```python
from build123d import *

# Parameters (mm, degrees)
SKETCH1_W               = 22
SKETCH1_H               = 52
BOSS_EXTRUDE1_DEPTH     = 9
CUT_EXTRUDE1_START      = 2
SKETCH2_W               = 20.1
SKETCH2_H               = 50.1
CUT_EXTRUDE1_DEPTH      = 10
SKETCH7_R               = 0.8
CUT_EXTRUDE6_DEPTH      = 9
CUT_EXTRUDE6_DEPTH_BACK = 2
CUT_EXTRUDE7_REACH      = 3
SKETCH8_R               = 1
CUT_EXTRUDE9_REACH      = 3
SKETCH9_R               = 1
CUT_EXTRUDE10_REACH     = 3
SKETCH10_R              = 1
CUT_EXTRUDE11_REACH     = 3
SKETCH11_R              = 1
CUT_EXTRUDE12_REACH     = 3
SKETCH12_R              = 1
CUT_EXTRUDE13_REACH     = 3
SKETCH13_R              = 1
CUT_EXTRUDE14_REACH     = 3
SKETCH14_R              = 1
CUT_EXTRUDE15_REACH     = 3
SKETCH15_R              = 1
CUT_EXTRUDE16_REACH     = 3
SKETCH16_R              = 1
SKETCH18_W              = 2.91
SKETCH18_H              = 52
BOSS_EXTRUDE2_DEPTH     = 2
SKETCH18_3_W            = 2.9
SKETCH18_3_H            = 52
BOSS_EXTRUDE3_DEPTH     = 2
SKETCH19_W              = 10
SKETCH19_H              = 7
CUT_EXTRUDE17_DEPTH     = 25.9
SKETCH20_W              = 3.86
SKETCH20_H              = 9.915252407
SKETCH20_W_2            = 4.307713093
CUT_EXTRUDE18_DEPTH     = 1


with BuildPart() as part:
    # Sketch1 → Boss-Extrude1 (new body)
    with BuildSketch(Plane(origin=(0, 0, 0), x_dir=(1, 0, 0), z_dir=(0, 1, 0))):
        Rectangle(SKETCH1_W, SKETCH1_H)
    extrude(amount=BOSS_EXTRUDE1_DEPTH)

    # Sketch2 → Cut-Extrude1 (cut)
    with BuildSketch(Plane(origin=(0, 9, 0), x_dir=(1, 0, 0), z_dir=(0, 1, 0)).offset(CUT_EXTRUDE1_START)):
        Rectangle(SKETCH2_W, SKETCH2_H)
    extrude(amount=-CUT_EXTRUDE1_DEPTH, mode=Mode.SUBTRACT)

    # Sketch7 → Cut-Extrude6 (cut, two sides)
    with BuildSketch(Plane(origin=(0, 1, 0), x_dir=(1, 0, 0), z_dir=(0, 1, 0))) as cut_extrude6_sk:
        with Locations((-8.15, -23)):
            Circle(SKETCH7_R)
    extrude(amount=CUT_EXTRUDE6_DEPTH, mode=Mode.SUBTRACT)
    extrude(cut_extrude6_sk.sketch, amount=-CUT_EXTRUDE6_DEPTH_BACK, mode=Mode.SUBTRACT)

    # Sketch8 → Cut-Extrude7 (cut, up to next)
    with BuildSketch(Plane(origin=(0, 1, 0), x_dir=(1, 0, 0), z_dir=(0, 1, 0)), mode=Mode.PRIVATE) as cut_extrude7_sk1:
        with Locations((-5.75, -12.3)):
            Circle(SKETCH8_R)
    cut_extrude7_tool1 = extrude(cut_extrude7_sk1.sketch, amount=-CUT_EXTRUDE7_REACH, mode=Mode.PRIVATE) & part.part
    add(cut_extrude7_tool1.solids().sort_by_distance((-5.75, 1, 12.3))[0], mode=Mode.SUBTRACT)
    # Sketch8 → Cut-Extrude7 (cut, up to next)
    with BuildSketch(Plane(origin=(0, 1, 0), x_dir=(1, 0, 0), z_dir=(0, 1, 0)), mode=Mode.PRIVATE) as cut_extrude7_sk2:
        with Locations((5, -12.3)):
            Circle(SKETCH8_R)
    cut_extrude7_tool2 = extrude(cut_extrude7_sk2.sketch, amount=-CUT_EXTRUDE7_REACH, mode=Mode.PRIVATE) & part.part
    add(cut_extrude7_tool2.solids().sort_by_distance((5, 1, 12.3))[0], mode=Mode.SUBTRACT)

    # Sketch9 → Cut-Extrude9 (cut, up to next)
    with BuildSketch(Plane(origin=(0, 1, 0), x_dir=(1, 0, 0), z_dir=(0, 1, 0)), mode=Mode.PRIVATE) as cut_extrude9_sk1:
        with Locations((-5.75, -9.5)):
            Circle(SKETCH9_R)
    cut_extrude9_tool1 = extrude(cut_extrude9_sk1.sketch, amount=-CUT_EXTRUDE9_REACH, mode=Mode.PRIVATE) & part.part
    add(cut_extrude9_tool1.solids().sort_by_distance((-5.75, 1, 9.5))[0], mode=Mode.SUBTRACT)
    # Sketch9 → Cut-Extrude9 (cut, up to next)
    with BuildSketch(Plane(origin=(0, 1, 0), x_dir=(1, 0, 0), z_dir=(0, 1, 0)), mode=Mode.PRIVATE) as cut_extrude9_sk2:
        with Locations((5, -9.5)):
            Circle(SKETCH9_R)
    cut_extrude9_tool2 = extrude(cut_extrude9_sk2.sketch, amount=-CUT_EXTRUDE9_REACH, mode=Mode.PRIVATE) & part.part
    add(cut_extrude9_tool2.solids().sort_by_distance((5, 1, 9.5))[0], mode=Mode.SUBTRACT)

    # Sketch10 → Cut-Extrude10 (cut, up to next)
    with BuildSketch(Plane(origin=(0, 1, 0), x_dir=(1, 0, 0), z_dir=(0, 1, 0)), mode=Mode.PRIVATE) as cut_extrude10_sk1:
        with Locations((-5.75, -6.8)):
            Circle(SKETCH10_R)
    cut_extrude10_tool1 = extrude(cut_extrude10_sk1.sketch, amount=-CUT_EXTRUDE10_REACH, mode=Mode.PRIVATE) & part.part
    add(cut_extrude10_tool1.solids().sort_by_distance((-5.75, 1, 6.8))[0], mode=Mode.SUBTRACT)
    # Sketch10 → Cut-Extrude10 (cut, up to next)
    with BuildSketch(Plane(origin=(0, 1, 0), x_dir=(1, 0, 0), z_dir=(0, 1, 0)), mode=Mode.PRIVATE) as cut_extrude10_sk2:
        with Locations((5, -6.837159935)):
            Circle(SKETCH10_R)
    cut_extrude10_tool2 = extrude(cut_extrude10_sk2.sketch, amount=-CUT_EXTRUDE10_REACH, mode=Mode.PRIVATE) & part.part
    add(cut_extrude10_tool2.solids().sort_by_distance((5, 1, 6.83716))[0], mode=Mode.SUBTRACT)

    # Sketch11 → Cut-Extrude11 (cut, up to next)
    with BuildSketch(Plane(origin=(0, 1, 0), x_dir=(1, 0, 0), z_dir=(0, 1, 0)), mode=Mode.PRIVATE) as cut_extrude11_sk1:
        with Locations((-0.3, -12.3)):
            Circle(SKETCH11_R)
    cut_extrude11_tool1 = extrude(cut_extrude11_sk1.sketch, amount=-CUT_EXTRUDE11_REACH, mode=Mode.PRIVATE) & part.part
    add(cut_extrude11_tool1.solids().sort_by_distance((-0.3, 1, 12.3))[0], mode=Mode.SUBTRACT)

    # Sketch12 → Cut-Extrude12 (cut, up to next)
    with BuildSketch(Plane(origin=(0, 1, 0), x_dir=(1, 0, 0), z_dir=(0, 1, 0)), mode=Mode.PRIVATE) as cut_extrude12_sk1:
        with Locations((3.95, 12.05)):
            Circle(SKETCH12_R)
    cut_extrude12_tool1 = extrude(cut_extrude12_sk1.sketch, amount=-CUT_EXTRUDE12_REACH, mode=Mode.PRIVATE) & part.part
    add(cut_extrude12_tool1.solids().sort_by_distance((3.95, 1, -12.05))[0], mode=Mode.SUBTRACT)
    # Sketch12 → Cut-Extrude12 (cut, up to next)
    with BuildSketch(Plane(origin=(0, 1, 0), x_dir=(1, 0, 0), z_dir=(0, 1, 0)), mode=Mode.PRIVATE) as cut_extrude12_sk2:
        with Locations((-6.8, 12.05)):
            Circle(SKETCH12_R)
    cut_extrude12_tool2 = extrude(cut_extrude12_sk2.sketch, amount=-CUT_EXTRUDE12_REACH, mode=Mode.PRIVATE) & part.part
    add(cut_extrude12_tool2.solids().sort_by_distance((-6.8, 1, -12.05))[0], mode=Mode.SUBTRACT)

    # Sketch13 → Cut-Extrude13 (cut, up to next)
    with BuildSketch(Plane(origin=(0, 1, 0), x_dir=(1, 0, 0), z_dir=(0, 1, 0)), mode=Mode.PRIVATE) as cut_extrude13_sk1:
        with Locations((3.95, 9.3)):
            Circle(SKETCH13_R)
    cut_extrude13_tool1 = extrude(cut_extrude13_sk1.sketch, amount=-CUT_EXTRUDE13_REACH, mode=Mode.PRIVATE) & part.part
    add(cut_extrude13_tool1.solids().sort_by_distance((3.95, 1, -9.3))[0], mode=Mode.SUBTRACT)
    # Sketch13 → Cut-Extrude13 (cut, up to next)
    with BuildSketch(Plane(origin=(0, 1, 0), x_dir=(1, 0, 0), z_dir=(0, 1, 0)), mode=Mode.PRIVATE) as cut_extrude13_sk2:
        with Locations((-6.8, 9.3)):
            Circle(SKETCH13_R)
    cut_extrude13_tool2 = extrude(cut_extrude13_sk2.sketch, amount=-CUT_EXTRUDE13_REACH, mode=Mode.PRIVATE) & part.part
    add(cut_extrude13_tool2.solids().sort_by_distance((-6.8, 1, -9.3))[0], mode=Mode.SUBTRACT)

    # Sketch14 → Cut-Extrude14 (cut, up to next)
    with BuildSketch(Plane(origin=(0, 1, 0), x_dir=(1, 0, 0), z_dir=(0, 1, 0)), mode=Mode.PRIVATE) as cut_extrude14_sk1:
        with Locations((3.9, 6.6)):
            Circle(SKETCH14_R)
    cut_extrude14_tool1 = extrude(cut_extrude14_sk1.sketch, amount=-CUT_EXTRUDE14_REACH, mode=Mode.PRIVATE) & part.part
    add(cut_extrude14_tool1.solids().sort_by_distance((3.9, 1, -6.6))[0], mode=Mode.SUBTRACT)
    # Sketch14 → Cut-Extrude14 (cut, up to next)
    with BuildSketch(Plane(origin=(0, 1, 0), x_dir=(1, 0, 0), z_dir=(0, 1, 0)), mode=Mode.PRIVATE) as cut_extrude14_sk2:
        with Locations((-6.85, 6.6)):
            Circle(SKETCH14_R)
    cut_extrude14_tool2 = extrude(cut_extrude14_sk2.sketch, amount=-CUT_EXTRUDE14_REACH, mode=Mode.PRIVATE) & part.part
    add(cut_extrude14_tool2.solids().sort_by_distance((-6.85, 1, -6.6))[0], mode=Mode.SUBTRACT)

    # Sketch15 → Cut-Extrude15 (cut, up to next)
    with BuildSketch(Plane(origin=(0, 1, 0), x_dir=(1, 0, 0), z_dir=(0, 1, 0)), mode=Mode.PRIVATE) as cut_extrude15_sk1:
        with Locations((-1.6, 11.05)):
            Circle(SKETCH15_R)
    cut_extrude15_tool1 = extrude(cut_extrude15_sk1.sketch, amount=-CUT_EXTRUDE15_REACH, mode=Mode.PRIVATE) & part.part
    add(cut_extrude15_tool1.solids().sort_by_distance((-1.6, 1, -11.05))[0], mode=Mode.SUBTRACT)

    # Sketch16 → Cut-Extrude16 (cut, up to next)
    with BuildSketch(Plane(origin=(0, 1, 0), x_dir=(1, 0, 0), z_dir=(0, 1, 0)), mode=Mode.PRIVATE) as cut_extrude16_sk1:
        with Locations((-8.25, 17.05)):
            Circle(SKETCH16_R)
    cut_extrude16_tool1 = extrude(cut_extrude16_sk1.sketch, amount=-CUT_EXTRUDE16_REACH, mode=Mode.PRIVATE) & part.part
    add(cut_extrude16_tool1.solids().sort_by_distance((-8.25, 1, -17.05))[0], mode=Mode.SUBTRACT)

    # Sketch18 → Boss-Extrude2 (add)
    with BuildSketch(Plane.XZ):
        with Locations((-12.455, 0)):
            Rectangle(SKETCH18_W, SKETCH18_H)
    extrude(amount=-BOSS_EXTRUDE2_DEPTH)

    # Sketch18<3> → Boss-Extrude3 (add)
    with BuildSketch(Plane.XZ):
        with Locations((12.45, -0.012983648)):
            Rectangle(SKETCH18_3_W, SKETCH18_3_H)
    extrude(amount=-BOSS_EXTRUDE3_DEPTH)

    # Sketch19 → Cut-Extrude17 (cut, through all)
    with BuildSketch(Plane.ZY.offset(11)):
        with Locations((0, 5.5)):
            Rectangle(SKETCH19_W, SKETCH19_H)
    extrude(amount=-CUT_EXTRUDE17_DEPTH, mode=Mode.SUBTRACT)

    # Sketch20 → Cut-Extrude18 (cut)
    with BuildSketch(Plane(origin=(0, 2, 0), x_dir=(1, 0, 0), z_dir=(0, 1, 0))):
        with Locations((-11.98, 0.042373796)):
            Rectangle(SKETCH20_W, SKETCH20_H)
        with Locations((12.203856547, 0.042373796)):
            Rectangle(SKETCH20_W_2, SKETCH20_H)
    extrude(amount=-CUT_EXTRUDE18_DEPTH, mode=Mode.SUBTRACT)


solid = part.part
```
Here's how the part is built. I have some questions about the finished solid (model axes, mm). A direction names the side the tool comes from. Coordinates: 2 decimals unless noted, no trailing zeros. Write each loop counter-clockwise with the first axis right and the second up, starting at its lowest first coordinate (ties: lowest second). Pieces come first, ordered by that corner, then holes. Notation, with made-up numbers: (66, 28) - (87, 28) arc R22 cw to (87, 58) - close; hole circle Ø7 at (67.25, 81.5). An arc over 180 degrees is marked (long way). One line per item, written item: value.
1) Suppose I cut it at B-B on z = -9.3. Write out the boundary of the cut face in (x, y), and give its area (3 significant figures).
Model answer:
outline: (-13.91, 0) - (-7.8, 0) - (-7.8, 1) - (-10.05, 1) - (-10.05, 9) - (-11, 9) - (-11, 2) - (-13.91, 2) - close; (-5.8, 0) - (2.95, 0) - (2.95, 1) - (-5.8, 1) - close; (4.95, 0) - (13.9, 0) - (13.9, 2) - (11, 2) - (11, 9) - (10.05, 9) - (10.05, 1) - (4.95, 1) - close
area: 44.8 mm²
2) On a 3-axis mill with a long thin cutter (end or side, diameter ignored), from which of +Z, -Z, +X, -X, +Y, -Y can I reach the whole of each face in a straight line? I mean faces 1 (the flat face through (-12, 2, -15)), 2 (the flat face through (12, 2, -15)), 3 (the flat face through (10.8, 3.8, -5)), 4 (the flat face through (0, 5, -25.05)), 5 (the cylindrical face through (4.87, 0.51, 11.31)). Say none if no direction works.
Model answer:
face 1: +Z, -Z, -X, +Y
face 2: +Z, -Z, +X, +Y
face 3: +X, -X, +Y
face 4: +Y
face 5: +Y, -Y
3) Suppose I cut it at D-D on y = 6. Write out the boundary of the cut face in (x, z), and give its area (3 significant figures).
Model answer:
outline: (-11, -26) - (11, -26) - (11, -5) - (10.05, -5) - (10.05, -25.05) - (-10.05, -25.05) - (-10.05, -5) - (-11, -5) - close; (-11, 5) - (-10.05, 5) - (-10.05, 25.05) - (10.05, 25.05) - (10.05, 5) - (11, 5) - (11, 26) - (-11, 26) - close
area: 118 mm²
4) I need wall thicknesses on line 1 along Z through (x, y) = (-8.15, 0.7); line 2 along Z through (x, y) = (-6.8, 0.7); line 3 along X through (y, z) = (0.35, 12.3). Which ranges of each line are inside material? Lowest first, please.
Model answer:
line 1: z = -26 to -18.04, -16.06 to 22.2, 23.8 to 26
line 2: z = -26 to -13.05, -11.05 to -10.3, -8.3 to -7.6, -5.6 to 26
line 3: x = -13.91 to -6.75, -4.75 to -1.3, 0.7 to 4, 6 to 13.9
5) I'm going to push flat-ended pins straight in: P1, Ø3, axis at x = -5.75, z = 12.3, coming from the +Y side; P2, Ø2.5, axis at x = -2, y = 6.5, coming from the -Z side; P3, Ø2.5, axis at y = 5, z = 15.5, coming from the +X side. Where does each tip first touch, or does it pass through?
Model answer:
P1: stops at y = 1
P2: stops at z = -26
P3: stops at x = 11
6) Suppose I cut it at C-C on x = 7.75. Write out the boundary of the cut face in (y, z), and give its area (3 significant figures).
Model answer:
outline: (0, -26) - (9, -26) - (9, -25.05) - (1, -25.05) - (1, 25.05) - (9, 25.05) - (9, 26) - (0, 26) - close
area: 67.2 mm²
